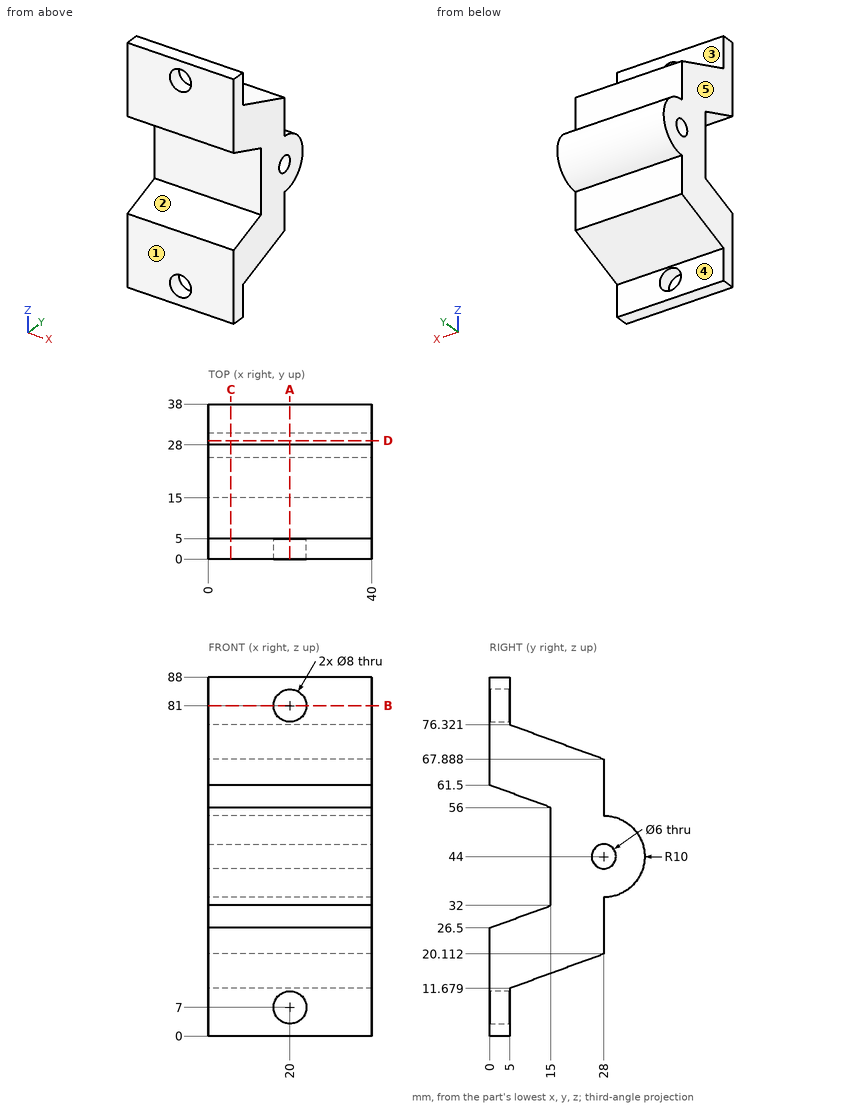
Answer from the drawing. Dimensions are ordinates in mm from the lowest x, y and z of the part. A direction names the side the tool comes from. Give positions to 0.01 mm unless a question says otherwise; leave off trailing zeros. Loops run counter-clockwise (first coordinate to the right, second up) from the corner with the lowest first, then second, coordinate; pieces in that order, holes last. Notation, with made-up numbers: (6, 68) -> (53, 68) arc R14 cw to (53, 85) -> close; hole circle Ø6 at (57.25, 60). An arc over 180 degrees is marked (long way). Answer as CSV lines item,"result".
Item 1: Find section C-C on x = 5.5. Give the vertices of the cut face in (y, z), plus the area to 3 significant figures.
Returned:
outline,"(0, 0) -> (5, 0) -> (5, 11.68) -> (28, 20.11) -> (28, 34) arc R10 ccw to (28, 54) -> (28, 67.89) -> (5, 76.32) -> (5, 88) -> (0, 88) -> (0, 61.5) -> (15, 56) -> (15, 32) -> (0, 26.5) -> close; hole circle Ø6 at (28, 44)"
area,"1,420 mm²"
Item 2: Find section B-B on z = 81. Give the vertices of the cut face in (x, y).
Returned:
outline,"(0, 0) -> (16, 0) -> (16, 5) -> (0, 5) -> close; (24, 0) -> (40, 0) -> (40, 5) -> (24, 5) -> close"
Item 3: Find section D-D on y = 29. Give the vertices of the cut face in (x, z).
Returned:
outline,"(0, 34.05) -> (40, 34.05) -> (40, 41.17) -> (0, 41.17) -> close; (0, 46.83) -> (40, 46.83) -> (40, 53.95) -> (0, 53.95) -> close"
Item 4: Each of these flat-tipped pins is pushed along its axis until it touches: pin 1 (1.5 mm diameter, centred on x = 22.5, y = 12, fed in from +Z); pin 2 (10 mm diameter, centred on x = 16.5, y = 27, fed in from +Z); pin 3 (5 mm diameter, centred on y = 28, z = 44, fed in from +X); pin 4 (4 mm diameter, centred on x = 27, z = 61.5, fed in from +Y). Where does it stop, or does it pass through?
Returned:
pin 1,"stops at z = 74.03"
pin 2,"stops at z = 70.09"
pin 3,"passes through"
pin 4,"stops at y = 28"
Item 5: For the marked faces 1, 2, 3, 4 and 5, determine the directions among +Z, -Z, +X, -X, +Y, -Y from which every point of the face is accessible in a straight line to the end or side of a thin tool.
Returned:
face 1,"+Z, -Z, +X, -X, -Y"
face 2,"+X, -X, -Y"
face 3,"+Z, +X, -X, +Y"
face 4,"-Z, +X, -X, +Y"
face 5,"+Z, -Z, -X, +Y, -Y"
Item 6: Find section A-A on x = 20. Give the vertices of the cut face in (y, z).
Returned:
outline,"(0, 0) -> (5, 0) -> (5, 3) -> (0, 3) -> close; (0, 11) -> (5, 11) -> (5, 11.68) -> (28, 20.11) -> (28, 34) arc R10 ccw to (28, 54) -> (28, 67.89) -> (5, 76.32) -> (5, 77) -> (0, 77) -> (0, 61.5) -> (15, 56) -> (15, 32) -> (0, 26.5) -> close; (0, 85) -> (5, 85) -> (5, 88) -> (0, 88) -> close; hole circle Ø6 at (28, 44)"
Item 7: Consider line 1 (X direction, y = 2, z = 7); line 2 (Y direction, x = 16.5, z = 44); line 3 (Z direction, x = 24, y = 30.5). Determine where each line is inside the solid, lowest interval first. Write a range as [from, to].
Returned:
line 1,"x = [0, 16], [24, 40]"
line 2,"y = [15, 25], [31, 38]"
line 3,"z = [34.32, 42.34], [45.66, 53.68]"
